The model under review builds one solid part; all positions refer to its coordinate system, in mm. Face numbers are marked on the shaded views. A direction names the side the tool comes from. Coordinates: 2 decimals unless noted, no trailing zeros. Write each loop counter-clockwise with the first axis right and the second up, starting at its lowest first coordinate (ties: lowest second). Pieces come first, ordered by that corner, then holes. Notation, with made-up numbers: M -1.75,83 L 5.25,83 A30 ccw 5.25,115 Z; hole C 28,-7.75 d10. An arc over 180 degrees is marked long. Answer as a JSON object with one key per item and string values.
Solid Edge part; units mm, degrees
sketch "Sketch1" plane through (0, 0, 0) normal (0, 0, 1) x (1, 0, 0)
  circle A0 centre (0, 0) radius 16.35
  line L0 (-12.4774, -1.6) -> (-10.3774, -1.6)
  line L1 (-12.4774, 0) -> (-12.4774, -1.6)
  line L2 (-12.4774, 0) -> (-12.4774, 1.6)
  line L3 (-12.4774, 1.6) -> (-10.3774, 1.6)
  arc A1 (-10.3774, 1.6) -> (-1.6, 10.3774) centre (0, 0) cw
  line L4 (-1.6, 12.4774) -> (-1.6, 10.3774)
  line L5 (0, 12.4774) -> (-1.6, 12.4774)
  line L6 (0, 12.4774) -> (1.6, 12.4774)
  line L7 (1.6, 12.4774) -> (1.6, 10.3774)
  arc A2 (1.6, 10.3774) -> (10.3774, 1.6) centre (0, 0) cw
  line L8 (12.4774, 1.6) -> (10.3774, 1.6)
  line L9 (12.4774, 0) -> (12.4774, 1.6)
  line L10 (12.4774, 0) -> (12.4774, -1.6)
  line L11 (12.4774, -1.6) -> (10.3774, -1.6)
  arc A3 (10.3774, -1.6) -> (1.6, -10.3774) centre (0, 0) cw
  line L12 (1.6, -12.4405) -> (1.6, -10.3774)
  line L13 (0, -12.4405) -> (1.6, -12.4405)
  line L14 (0, -12.4405) -> (-1.6, -12.4405)
  line L15 (-1.6, -12.4405) -> (-1.6, -10.3774)
  arc A4 (-1.6, -10.3774) -> (-10.3774, -1.6) centre (0, 0) cw
extrude "Protrusion1" add sketch "Sketch1" along normal blind 16.2
sketch "Sketch2" plane through (0, 0, 16.2) normal (0, 0, 1) x (1, 0, 0)
  circle A0 centre (0, 0) radius 14.75
  circle A1 centre (0, 0) radius 17.5589
extrude "ScavoEstrusione_1" cut sketch "Sketch2" against normal blind 11.3
chamfer "Smusso_1" distance 0.5 angle 45 1 edges at (-14.75, 0, 16.2)
fillet "Rotondo_1" radius 0.4 1 edges at (-14.75, 0, 4.9)
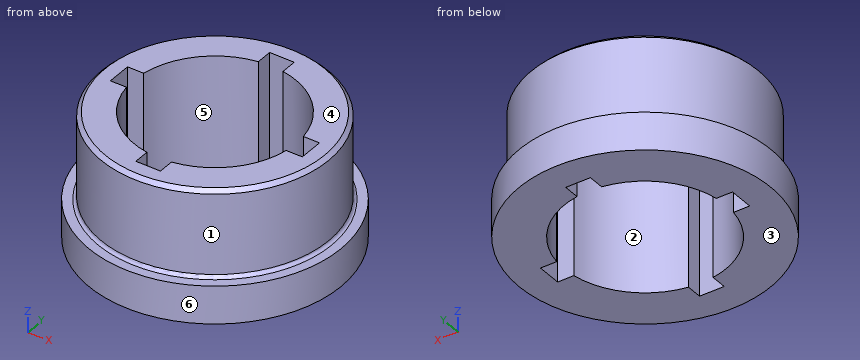
(1) Add section A-A on z = 12. Give the boundary of the cut face in (x, y).
Results list:
{"outline": "C 0,0 d29.5; hole M -12.48,-1.6 L -10.38,-1.6 A10.5 ccw -1.6,-10.38 L -1.6,-12.44 L 1.6,-12.44 L 1.6,-10.38 A10.5 ccw 10.38,-1.6 L 12.48,-1.6 L 12.48,1.6 L 10.38,1.6 A10.5 ccw 1.6,10.38 L 1.6,12.48 L -1.6,12.48 L -1.6,10.38 A10.5 ccw -10.38,1.6 L -12.48,1.6 Z"}
(2) For the marked faces 1, 2 and 3, list the 3-axis set-ups (+Z, -Z, +X, -X, +Y, -Y) from which the entire face can be reached by the end or side of a thin tool; tool diameter is ignored.
Results list:
{"face 1": "+Z", "face 2": "+Z, -Z", "face 3": "-Z, +X, -X, +Y, -Y"}
(3) Add section C-C on y = 0. Give the boundary of the cut face in (x, z), and give its area (3 significant figures).
Results list:
{"outline": "M -16.35,0 L -12.48,0 L -12.48,16.2 L -14.25,16.2 L -14.75,15.7 L -14.75,5.3 A0.4 cw -15.15,4.9 L -16.35,4.9 Z; M 12.48,0 L 16.35,0 L 16.35,4.9 L 15.15,4.9 A0.4 cw 14.75,5.3 L 14.75,15.7 L 14.25,16.2 L 12.48,16.2 Z", "area": "89.1 mm²"}
(4) For pin 1 Ø0.6 at (y, z) = (11, 5) entering from +X; pin 2 Ø1.1 at (x, z) = (12, 7.5) entering from +Y; pin 3 Ø0.6 at (x, z) = (-11, 9) entering from -Y, all flat-tipped, find the tip position at first contact; note any pin that passes through.
Results list:
{"pin 1": "x = 12.35", "pin 2": "y = 9.3", "pin 3": "y = -10.15"}
(5) Add section B-B on x = 0. Give the boundary of the cut face in (y, z).
Results list:
{"outline": "M -16.35,0 L -12.44,0 L -12.44,16.2 L -14.25,16.2 L -14.75,15.7 L -14.75,5.3 A0.4 cw -15.15,4.9 L -16.35,4.9 Z; M 12.48,0 L 16.35,0 L 16.35,4.9 L 15.15,4.9 A0.4 cw 14.75,5.3 L 14.75,15.7 L 14.25,16.2 L 12.48,16.2 Z"}
(6) Add section D-D on z = 3.25. Give the boundary of the cut face in (x, y).
Results list:
{"outline": "C 0,0 d32.7; hole M -12.48,-1.6 L -10.38,-1.6 A10.5 ccw -1.6,-10.38 L -1.6,-12.44 L 1.6,-12.44 L 1.6,-10.38 A10.5 ccw 10.38,-1.6 L 12.48,-1.6 L 12.48,1.6 L 10.38,1.6 A10.5 ccw 1.6,10.38 L 1.6,12.48 L -1.6,12.48 L -1.6,10.38 A10.5 ccw -10.38,1.6 L -12.48,1.6 Z"}
(7) Wall thickness on line 1 along Y through (x, z) = (0.5, 14.5); line 2 along X through (y, z) = (-0.5, 3.25); line 3 along X through (y, z) = (12, 9.25): over which ranges is each line inside the solid? List them lowest first. Write a range as from..to.
Results list:
{"line 1": "-14.74..-12.44, 12.48..14.74", "line 2": "-16.34..-12.48, 12.48..16.34", "line 3": "-8.58..-1.6, 1.6..8.58"}
(8) Draft analysis for pull direction Y (two halves, no side actions). For the marked faces 4, 5 and 6, state which applies: released by +Y, released by -Y, zero draft, split by the parting line, or undercut.
Results list:
{"face 4": "zero draft", "face 5": "undercut", "face 6": "split by the parting line"}
